Autodesk Inventor part; units mm, degrees
ref_plane "YZ Plane" through (0, 0, 0) normal (1, 0, 0) x (0, 1, 0)
ref_plane "XZ Plane" through (0, 0, 0) normal (0, 1, 0) x (-1, 0, 0)
ref_plane "XY Plane" through (0, 0, 0) normal (0, 0, 1) x (1, 0, 0)
sketch "Эскиз1" plane through (0, 0, 0) normal (1, 0, 0) x (0, 1, 0)
  point P0 (0, 0)
sketch "Эскиз2" plane through (0, 0, 0) normal (0, 1, 0) x (-1, 0, 0)
  line L0 (19, -4) -> (-19, -4)
  line L1 (-19, -4) -> (-19, 4)
  line L2 (-19, 4) -> (19, 4)
  line L3 (19, 4) -> (19, -4)
  line L4 (19, -4) -> (-19, 4) construction
  line L5 (-19, -4) -> (19, 4) construction
  line L6 (19, 0) -> (-19, 0) construction
  circle A0 centre (-15, 0) radius 1.5
  line L7 (0, -4) -> (0, 4) construction
  circle A1 centre (15, 0) radius 1.5
  point P0 (0, 0)
  dimension "d1" = 30
  dimension "d2" = 3
  dimension "d3" = 38
  dimension "d4" = 8
extrude "Выдавливание1" add sketch "Эскиз2" along normal blind 35
fillet "Сопряжение1" radius 3.5 4 edges at (19, 17.5, 4) (19, 17.5, -4) (-19, 17.5, 4) (-19, 17.5, -4)
sketch "Эскиз3" plane through (-15.5, 0, 4) normal (0, 0, 1) x (1, 0, 0)
  line L0 (29, 35) -> (29, 0) construction
  line L1 (0, 0) -> (0, 35) construction
  line L2 (0, 0) -> (31, 0) construction
  line L3 (31, 35) -> (31, 0) construction
  line L4 (0, 35) -> (31, 35) construction
  line L5 (32, 35) -> (32, 0) construction
  line L6 (34.5, 35) -> (31, 35) construction
  line L7 (31, 35) -> (31, 0) construction
  line L8 (31, 0) -> (34.5, 0) construction
  line L9 (34.5, 0) -> (34.5, 35) construction
  line L10 (-1, 35) -> (-1, 0) construction
  line L11 (0, 35) -> (-3.5, 35) construction
  line L12 (-3.5, 35) -> (-3.5, 0) construction
  line L13 (-3.5, 0) -> (0, 0) construction
  line L14 (0, 0) -> (0, 35) construction
  line L15 (0, 0) -> (0, 35) construction
  line L16 (-1, 35) -> (2, 35) construction
  line L17 (29, 35) -> (32, 35) construction
  line L18 (29, 0) -> (32, 0) construction
  line L19 (-1, 35) -> (2, 35) construction
  line L20 (-1, 0) -> (2, 0) construction
  line L21 (-1, 35) -> (2, 35) construction
  line L22 (-1, 0) -> (2, 0) construction
  line L23 (2, 35) -> (2, 0) construction
  line L24 (29, 35) -> (2, 0) construction
  line L25 (2, 35) -> (29, 0) construction
  line L26 (15.5, 17.5) -> (15.5, 35) construction
  line L27 (0, 35) -> (31, 35) construction
  circle A0 centre (15.5, 12) radius 10.5
  point P0 (15.5, 0)
  dimension "d8" = 21
  dimension "d9" = 12
extrude "Выдавливание2" cut sketch "Эскиз3" against normal blind 35
properties part number "mid_mount" material "Пластик АБС"
CAD build for the part. Positions are in the model's coordinates, mm. Give positions to 0.01 mm unless a question says otherwise; leave off trailing zeros. Write each loop counter-clockwise with the first axis right and the second up, starting at its lowest first coordinate (ties: lowest second). Pieces come first, ordered by that corner, then holes. Notation, with made-up numbers: M 81,53 L 139,53 A34 cw 139,92 Z; hole C -19,63 d9. An arc over 180 degrees is marked long. Put each result on its own line as item: value. Start each with the question number.
(1) Band-saw the part on B-B, the plane y = 12. Write the cut outline in (x, z).
(2) Flat gauge pin, fed straight in: pin 1 Ø1.5 at (y, z) = (29.5, 2.5) entering from +X. Where does the tip first touch, or does it go through?
(3) Probe L1, parallel to X at y = 21.5, z = -1.25; L2, parallel to X at y = 18.5, z = 0.5; L3, parallel to X at y = 32.5, z = -1. List the from-to ranges inside material, lowest first.
(4) Band-saw the part on C-C, the plane x = 15. Write the cut outline in (y, z).
(5) Band-saw the part on A-A, the plane z = 0. Write the cut outline in (x, y).
(6) Band-saw the part on D-D, the plane x = 0. Write the cut outline in (y, z), and give its area (3 significant figures).
(7) Mould opens along X. For faces 1 (the face through (0, 35, 0)), 2 (the face through (5.645, 20.854, 0.056)), 3 (the face through (17.95, 17.74, 3)), 4 (the face through (16.5, 17.26, -0.07)) say: +X half, -X half, draft (parallel to the pull), parting line (faces both ways), or undercut.
Response values:
1. outline: M -19,-0.5 A3.5 ccw -15.5,-4 L -10.5,-4 L -10.5,4 L -15.5,4 A3.5 ccw -19,0.5 Z; M 10.5,-4 L 15.5,-4 A3.5 ccw 19,-0.5 L 19,0.5 A3.5 ccw 15.5,4 L 10.5,4 Z; hole C -15,0 d3; hole C 15,0 d3
2. pin 1: stops at x = 18.77
3. L1: x = -18.92 to -15.83, -14.17 to -4.47, 4.47 to 14.17, 15.83 to 18.92
3. L2: x = -19 to -16.41, -13.59 to -8.25, 8.25 to 13.59, 16.41 to 19
3. L3: x = -18.96 to -16.12, -13.88 to 13.88, 16.12 to 18.96
4. outline: M 0,-4 L 35,-4 L 35,-1.5 L 0,-1.5 Z; M 0,1.5 L 35,1.5 L 35,4 L 0,4 Z
5. outline: M -19,0 L -16.5,0 L -16.5,35 L -19,35 Z; M -13.5,0 L 13.5,0 L 13.5,35 L -13.5,35 Z; M 16.5,0 L 19,0 L 19,35 L 16.5,35 Z; hole C 0,12 d21
6. outline: M 0,-4 L 1.5,-4 L 1.5,4 L 0,4 Z; M 22.5,-4 L 35,-4 L 35,4 L 22.5,4 Z
6. area: 112 mm2
7. face 1: draft
7. face 2: undercut
7. face 3: +X half
7. face 4: undercut
